Answer from the drawing. Dimensions are ordinates in mm from the lowest x, y and z of the part. A direction names the side the tool comes from. Give positions to 0.01 mm unless a question says otherwise; leave off trailing zeros. Loops run counter-clockwise (first coordinate to the right, second up) from the corner with the lowest first, then second, coordinate; pieces in that order, holes last. Notation, with made-up numbers: (-8, 43.5) - (28, 43.5) arc R13 cw to (28, 60.5) - close; hole circle Ø8 at (-19.75, 4). An arc over 180 degrees is marked (long way). One line per item, written item: value.
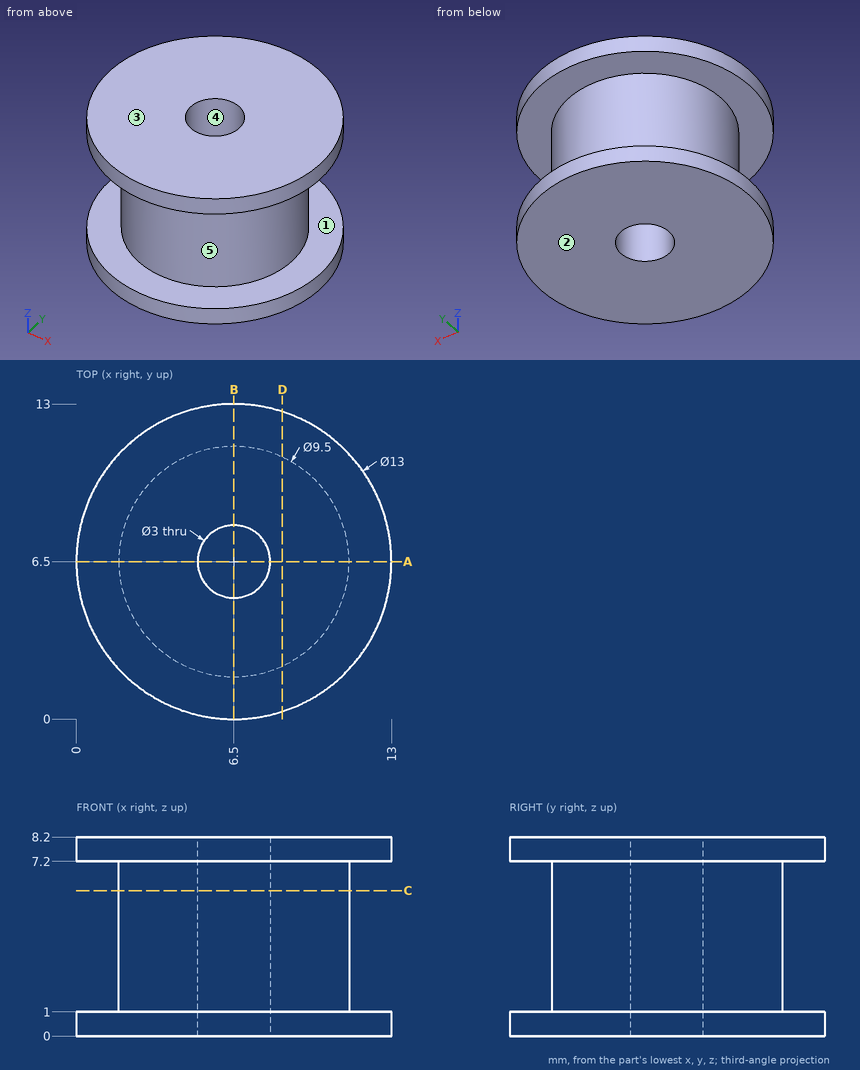
1. Section C-C (z = 6) is taken. Write down the section's boundary in (x, y).
Output:
outline: circle Ø9.5 at (6.5, 6.5); hole circle Ø3 at (6.5, 6.5)
2. A flat-ended cylindrical pin translates along its axis: pin 1 Ø4 at (x, z) = (2, 7) entering from +Y. Find the tip coordinate at first contact, or state that the pin passes through.
Output:
pin 1: stops at y = 12.5
3. Section D-D (x = 8.5) is taken. Write down the section's boundary in (y, z), and give its area (3 significant figures).
Output:
outline: (0.32, 0) - (12.68, 0) - (12.68, 1) - (10.81, 1) - (10.81, 7.2) - (12.68, 7.2) - (12.68, 8.2) - (0.32, 8.2) - (0.32, 7.2) - (2.19, 7.2) - (2.19, 1) - (0.32, 1) - close
area: 78.2 mm²
4. The mould has two halves that part along X. Classify the marked faces 3, 4 and 5: released by +X, released by -X, zero draft, split by the parting line, or undercut.
Output:
face 3: zero draft
face 4: undercut
face 5: split by the parting line
5. Find the intervals of material crossed by line 1 along Y through (x, z) = (6.5, 2.5); line 2 along Z through (x, y) = (1.5, 5.25); line 3 along X through (y, z) = (7.5, 6.5), in increasing order.
Output:
line 1: y = 1.75 to 5, 8 to 11.25
line 2: z = 0 to 1, 7.2 to 8.2
line 3: x = 1.86 to 5.38, 7.62 to 11.14
6. Section A-A (y = 6.5) is taken. Write down the section's boundary in (x, z).
Output:
outline: (0, 0) - (5, 0) - (5, 8.2) - (0, 8.2) - (0, 7.2) - (1.75, 7.2) - (1.75, 1) - (0, 1) - close; (8, 0) - (13, 0) - (13, 1) - (11.25, 1) - (11.25, 7.2) - (13, 7.2) - (13, 8.2) - (8, 8.2) - close
7. For the marked faces 1 and 2, determine the directions among +Z, -Z, +X, -X, +Y, -Y from which every point of the face is accessible in a straight line to the end or side of a thin tool.
Output:
face 1: none
face 2: -Z, +X, -X, +Y, -Y
